Check sheet for the modelled part. Datum: model origin and axes. Units: mm. Face numbers are marked on the shaded views. A direction names the side the tool comes from. Round coordinates to 2 decimals unless told otherwise and drop trailing zeros. Order: outer loops, then holes, each group sorted by start corner. A loop starts at its lowest first (then second) coordinate and runs counter-clockwise, first axis right, second up.
Q1. Set-up check for the marked faces 1 and 2: record each of +Z, -Z, +X, -X, +Y, -Y from which the full face is reachable in a straight line by a thin tool's end or side.
Q2. Cross-section at B-B on x = 45. Record the cut outline in (y, z).
Q3. Depth check by flat-ended pin: P1, Ø3, axis at x = 15, z = -38, coming from the +Y side; P2, Ø14, axis at x = -1, z = -12.5, coming from the -Y side; P3, Ø5.5, axis at x = -18, y = -35.18, coming from the -Z side. Enter the tip coordinate at first touch or a pass-through.
Q4. Scan lines: probe 1 along X at (y, z) = (43.4, -38); probe 2 along X at (y, z) = (-35, 1); probe 3 along X at (y, z) = (32, 1.65). Record each from-to range of solid material in increasing order.
Q5. Cross-section at D-D on z = -3. Record the cut outline in (x, y), then the cut area to 3 significant figures.
Q6. Cross-section at C-C on y = 32. Record the cut outline in (x, z), then the cut area to 3 significant figures.
Q7. Cross-section at A-A on z = -31. Record the cut outline in (x, y), then the cut area to 3 significant figures.
Autodesk Inventor part; units mm, degrees
ref_plane "YZ Plane" through (0, 0, 0) normal (1, 0, 0) x (0, 1, 0)
ref_plane "XZ Plane" through (0, 0, 0) normal (0, 1, 0) x (-1, 0, 0)
ref_plane "XY Plane" through (0, 0, 0) normal (0, 0, 1) x (1, 0, 0)
sketch "Sketch3" plane through (0, 0, 0) normal (0, 0, 1) x (1, 0, 0)
  line L0 (-50, 45) -> (50, 45)
  line L1 (50, 45) -> (50, -45)
  line L2 (50, -45) -> (-50, -45)
  line L3 (-50, -45) -> (-50, 45)
  line L4 (-50, 45) -> (50, -45) construction
  line L5 (50, 45) -> (-50, -45) construction
  point P0 (0, 0)
  dimension "d4" = 100
  dimension "d5" = 90
extrude "Extrusion2" add sketch "Sketch3" along normal blind 4
sketch "Sketch4" plane through (0, 0, 4) normal (0, 0, 1) x (1, 0, 0)
  point P0 (0, 0)
sketch "Sketch5" plane through (0, 0, 4) normal (0, 0, 1) x (1, 0, 0)
  line L0 (50, 45) -> (-50, 45)
  line L1 (50, 45) -> (-50, 45)
  line L2 (-50, 45) -> (-50, 41)
  line L3 (-50, 41) -> (50, 41)
  line L4 (50, 41) -> (50, 45)
  point P0 (0, 0)
  dimension "d8" = 4
  dimension "d9" = 100
extrude "Extrusion3" add sketch "Sketch5" against normal blind 50
sketch "Sketch6" plane through (0, 0, 4) normal (0, 0, 1) x (1, 0, 0)
  line L0 (18, -31.18) -> (-18, -31.18)
  line L1 (-18, -31.18) -> (-18, 31.18)
  line L2 (-18, 31.18) -> (18, 31.18)
  line L3 (18, 31.18) -> (18, -31.18)
  line L4 (18, -31.18) -> (-18, 31.18) construction
  line L5 (-18, -31.18) -> (18, 31.18) construction
  circle A0 centre (-18, 31.18) radius 1.75
  circle A1 centre (18, 31.18) radius 1.75
  circle A2 centre (-18, -31.18) radius 1.75
  circle A3 centre (18, -31.18) radius 1.75
  line L6 (50, 45) -> (-50, 45)
  line L7 (0, 45) -> (0, -4)
  line L8 (-18, -35.18) -> (18, -35.18)
  line L9 (18, -35.18) -> (18, 27.18)
  line L10 (18, 27.18) -> (-18, 27.18)
  line L11 (-18, 27.18) -> (-18, -35.18)
  line L12 (-18, -35.18) -> (18, 27.18) construction
  line L13 (18, -35.18) -> (-18, 27.18) construction
  circle A4 centre (18, 27.18) radius 1.75
  circle A5 centre (-18, 27.18) radius 1.75
  circle A6 centre (18, -35.18) radius 1.75
  circle A7 centre (-18, -35.18) radius 1.75
  point P0 (0, 0)
  dimension "d14" = 3.5
  dimension "d15" = 3.5
  dimension "d16" = 3.5
  dimension "d17" = 3.5
  dimension "d89" = 49
  dimension "d90" = 62.36
  dimension "d91" = 3.5
  dimension "d92" = 3.5
  dimension "d93" = 3.5
  dimension "d94" = 3.5
extrude "Extrusion4" cut sketch "Sketch6" against normal blind 50 contours A5 L1 | L1 L10 A5 | A7 L8 L11 | L11 L8 A7 | A4 L10 L3 | L3 A4 | A6 L8 L9 | L9 L8 A6 | L1 A5 L10 | L10 A4 L3
sketch "Sketch7" plane through (0, 0, 4) normal (0, 0, 1) x (1, 0, 0)
  line L0 (31.18, -18) -> (-31.18, -18)
  line L1 (-31.18, -18) -> (-31.18, 18)
  line L2 (-31.18, 18) -> (31.18, 18)
  line L3 (31.18, 18) -> (31.18, -18)
  line L4 (31.18, -18) -> (-31.18, 18) construction
  line L5 (-31.18, -18) -> (31.18, 18) construction
  circle A0 centre (-31.18, 18) radius 1.75
  circle A1 centre (31.18, 18) radius 1.75
  circle A2 centre (-31.18, -18) radius 1.75
  circle A3 centre (31.18, -18) radius 1.75
  line L6 (50, 45) -> (-50, 45)
  line L7 (0, 45) -> (0, -4)
  line L8 (-31.18, -22) -> (31.18, -22)
  line L9 (31.18, -22) -> (31.18, 14)
  line L10 (31.18, 14) -> (-31.18, 14)
  line L11 (-31.18, 14) -> (-31.18, -22)
  line L12 (-31.18, -22) -> (31.18, 14) construction
  line L13 (31.18, -22) -> (-31.18, 14) construction
  circle A4 centre (31.18, 14) radius 1.75
  circle A5 centre (-31.18, 14) radius 1.75
  circle A6 centre (31.18, -22) radius 1.75
  circle A7 centre (-31.18, -22) radius 1.75
  point P0 (0, 0)
  dimension "d20" = 62.36
  dimension "d21" = 36
  dimension "d22" = 3.5
  dimension "d23" = 3.5
  dimension "d24" = 3.5
  dimension "d25" = 3.5
  dimension "d95" = 49
  dimension "d96" = 36
  dimension "d97" = 3.5
  dimension "d98" = 3.5
  dimension "d99" = 3.5
  dimension "d100" = 3.5
extrude "Extrusion5" cut sketch "Sketch7" against normal blind 50 contours A5 L1 | L1 L10 A5 | A7 L8 L11 | L11 L8 A7 | A4 L10 L3 | L3 A4 | A6 L8 L9 | L9 L8 A6 | L1 A5 L10 | L10 A4 L3
sketch "Sketch8" plane through (0, 0, 4) normal (0, 0, 1) x (1, 0, 0)
  line L0 (50, 45) -> (-50, 45)
  line L1 (0, 45) -> (0, -4)
  circle A0 centre (0, -4) radius 25
  point P0 (0, 0)
  dimension "d101" = 49
  dimension "d102" = 50
extrude "Extrusion6" cut sketch "Sketch8" against normal blind 43.6625
sketch "Sketch9" plane through (-50, 45, 4) normal (0, 1, 0) x (1, 0, 0)
  line L0 (0, 50) -> (0, 0)
  line L1 (100, 0) -> (0, 0)
  line L2 (0, 0) -> (35, 0)
  line L3 (35, 0) -> (35, 7)
  line L4 (35, 7) -> (0, 7)
  line L5 (0, 7) -> (0, 0)
  circle A0 centre (35, 7) radius 1.75
  line L6 (0, 0) -> (35, 0)
  line L7 (35, 0) -> (35, 25)
  line L8 (35, 25) -> (0, 25)
  line L9 (0, 25) -> (0, 0)
  circle A1 centre (35, 25) radius 1.75
  point P0 (50, 4)
  dimension "d31" = 35
  dimension "d32" = 7
  dimension "d36" = 3.5
  dimension "d39" = 25
  dimension "d40" = 3.5
sketch "Sketch10" plane through (-50, 45, 4) normal (0, 1, 0) x (1, 0, 0)
  line L0 (100, 4) -> (100, 0)
  line L1 (100, 0) -> (0, 0)
  line L2 (100, 0) -> (65, 0)
  line L3 (65, 0) -> (65, 7)
  line L4 (65, 7) -> (100, 7)
  line L5 (100, 7) -> (100, 0)
  circle A0 centre (65, 7) radius 1.75
  line L6 (100, 0) -> (65, 0)
  line L7 (65, 0) -> (65, 25)
  line L8 (65, 25) -> (100, 25)
  line L9 (100, 25) -> (100, 0)
  line L10 (75, 0) -> (25, 0)
  circle A1 centre (65, 25) radius 1.75
  point P0 (50, 4)
  dimension "d33" = 35
  dimension "d34" = 7
  dimension "d35" = 3.5
  dimension "d37" = 25
  dimension "d38" = 3.5
sketch "Sketch11" plane through (-50, 45, 4) normal (0, 1, 0) x (1, 0, 0)
  point P0 (50, 4)
extrude "Extrusion7" cut sketch "Sketch9" against normal blind 43.6625 contours A1 L7 L8 | L8 L7 A1 | A0 L7 L4 | L4 L3 A0 | L7 A0 L3
extrude "Extrusion8" cut sketch "Sketch10" against normal blind 43.6625 contours A0 L3 L4 | L4 L7 A0 | L3 A0 L7 | A1 L7 L8 | L8 L7 A1
sketch "Sketch12" plane through (-50, 45, 4) normal (0, 1, 0) x (1, 0, 0)
  line L0 (0, 0) -> (100, 0)
  line L1 (0, 0) -> (5, 0)
  line L2 (5, 0) -> (5, 7)
  line L3 (5, 7) -> (0, 7)
  line L4 (0, 7) -> (0, 0)
  line L5 (100, 0) -> (0, 0)
  line L6 (0, 0) -> (5, 0)
  line L7 (5, 0) -> (5, 25)
  line L8 (5, 25) -> (0, 25)
  line L9 (0, 25) -> (0, 0)
  circle A0 centre (5, 7) radius 1.75
  circle A1 centre (5, 25) radius 1.75
  point P0 (50, 4)
  dimension "d45" = 5
  dimension "d46" = 7
  dimension "d47" = 25
  dimension "d48" = 3.5
  dimension "d49" = 3.5
extrude "Extrusion9" cut sketch "Sketch12" against normal blind 43.6625 contours A0 L3 L2 | L2 L7 A0 | A0 L7 L3 | A1 L7 L8 | L8 L7 A1
sketch "Sketch13" plane through (-50, 45, 4) normal (0, 1, 0) x (1, 0, 0)
  line L0 (0, 0) -> (100, 0)
  line L1 (100, 0) -> (95, 0)
  line L2 (95, 0) -> (95, 7)
  line L3 (95, 7) -> (100, 7)
  line L4 (100, 7) -> (100, 0)
  line L5 (100, 0) -> (95, 0)
  line L6 (95, 0) -> (95, 25)
  line L7 (95, 25) -> (100, 25)
  line L8 (100, 25) -> (100, 0)
  circle A0 centre (95, 25) radius 1.75
  circle A1 centre (95, 7) radius 1.75
  point P0 (50, 4)
  dimension "d52" = 5
  dimension "d53" = 7
  dimension "d54" = 25
  dimension "d55" = 3.5
  dimension "d56" = 3.5
extrude "Extrusion10" cut sketch "Sketch13" against normal blind 43.6625 contours A1 L6 L2 | L2 L3 A1 | L6 A1 L3 | A0 L7 L6 | L6 L7 A0
sketch "Sketch14" plane through (-50, 45, 4) normal (0, 1, 0) x (1, 0, 0)
  point P0 (50, 4)
sketch "Sketch15" plane through (-50, 45, 4) normal (0, 1, 0) x (1, 0, 0)
  line L0 (0, 50) -> (100, 50)
  line L1 (0, 50) -> (50, 50)
  line L2 (50, 50) -> (50, 42)
  line L3 (50, 42) -> (0, 42)
  line L4 (0, 42) -> (0, 50)
  line L5 (0, 50) -> (35, 50)
  line L6 (35, 50) -> (35, 42)
  line L7 (35, 42) -> (0, 42)
  line L8 (0, 42) -> (0, 50)
  line L9 (0, 4) -> (0, 50)
  line L10 (0, 50) -> (5, 50)
  line L11 (5, 50) -> (5, 42)
  line L12 (5, 42) -> (0, 42)
  line L13 (0, 42) -> (0, 50)
  line L14 (100, 4) -> (100, 50)
  line L15 (100, 50) -> (95, 50)
  line L16 (95, 50) -> (95, 42)
  line L17 (95, 42) -> (100, 42)
  line L18 (100, 42) -> (100, 50)
  line L19 (100, 50) -> (0, 50)
  line L20 (100, 50) -> (65, 50)
  line L21 (65, 50) -> (65, 42)
  line L22 (65, 42) -> (100, 42)
  line L23 (100, 42) -> (100, 50)
  circle A0 centre (5, 42) radius 1.75
  circle A1 centre (35, 42) radius 1.75
  circle A2 centre (65, 42) radius 1.75
  circle A3 centre (95, 42) radius 1.75
  point P0 (50, 4)
  dimension "d60" = 8
  dimension "d61" = 35
  dimension "d62" = 5
  dimension "d63" = 5
  dimension "d64" = 35
  dimension "d66" = 3.5
  dimension "d67" = 3.5
  dimension "d68" = 3.5
  dimension "d69" = 3.5
extrude "Extrusion11" cut sketch "Sketch15" against normal blind 43.6625 contours A0 L3 L11 | L11 L3 A0 | L3 A0 | A1 L3 L6 | L6 L3 A1 | L3 A1 | A2 L22 L21 | L21 L22 A2 | A3 L17 L16 | L16 L22 A3 | L17 A3 L22
sketch "Sketch16" plane through (-50, 45, 4) normal (0, 1, 0) x (1, 0, 0)
  line L0 (100, 50) -> (0, 50)
  line L1 (0, 50) -> (20, 50)
  line L2 (20, 50) -> (20, 35)
  line L3 (20, 35) -> (0, 35)
  line L4 (0, 35) -> (0, 50)
  line L5 (0, 50) -> (0, 0)
  line L6 (0, 50) -> (50, 50)
  line L7 (50, 50) -> (50, 35)
  line L8 (50, 35) -> (0, 35)
  line L9 (0, 35) -> (0, 50)
  line L10 (100, 4) -> (100, 50)
  line L11 (100, 50) -> (80, 50)
  line L12 (80, 50) -> (80, 35)
  line L13 (80, 35) -> (100, 35)
  line L14 (100, 35) -> (100, 50)
  circle A0 centre (20, 35) radius 1.75
  circle A1 centre (50, 35) radius 1.75
  circle A2 centre (80, 35) radius 1.75
  point P0 (50, 4)
  dimension "d72" = 20
  dimension "d73" = 15
  dimension "d74" = 50
  dimension "d75" = 20
  dimension "d76" = 3.5
  dimension "d77" = 3.5
  dimension "d78" = 3.5
extrude "Extrusion12" cut sketch "Sketch16" against normal blind 10 contours A2 L13 L12 | L12 L13 A2 | A1 L8 L7 | L7 L8 A1 | A0 L8 L2 | L2 L3 A0 | L8 A0 L3
sketch "Sketch17" plane through (0, 0, 4) normal (0, 0, 1) x (1, 0, 0)
  line L0 (36, -36) -> (-36, -36)
  line L1 (-36, -36) -> (-36, 36)
  line L2 (-36, 36) -> (36, 36)
  line L3 (36, 36) -> (36, -36)
  line L4 (36, -36) -> (-36, 36) construction
  line L5 (-36, -36) -> (36, 36) construction
  circle A0 centre (-36, 36) radius 1.75
  circle A1 centre (36, 36) radius 1.75
  circle A2 centre (36, -36) radius 1.75
  circle A3 centre (-36, -36) radius 1.75
  line L6 (50, 45) -> (-50, 45)
  line L7 (0, 45) -> (0, -4)
  line L8 (-36, -40) -> (36, -40)
  line L9 (36, -40) -> (36, 32)
  line L10 (36, 32) -> (-36, 32)
  line L11 (-36, 32) -> (-36, -40)
  line L12 (-36, -40) -> (36, 32) construction
  line L13 (36, -40) -> (-36, 32) construction
  circle A4 centre (36, 32) radius 1.75
  circle A5 centre (36, -40) radius 1.75
  circle A6 centre (-36, -40) radius 1.75
  circle A7 centre (-36, 32) radius 1.75
  point P0 (0, 0)
  dimension "d81" = 72
  dimension "d82" = 72
  dimension "d83" = 3.5
  dimension "d84" = 3.5
  dimension "d85" = 3.5
  dimension "d86" = 3.5
  dimension "d103" = 49
  dimension "d104" = 72
  dimension "d105" = 3.5
  dimension "d106" = 3.5
  dimension "d107" = 3.5
  dimension "d108" = 3.5
extrude "Extrusion13" cut sketch "Sketch17" against normal blind 10 contours A7 L1 | L1 L10 A7 | A6 L8 L11 | L11 L8 A6 | A4 L10 L3 | L3 A4 | A5 L8 L9 | L9 L8 A5 | L1 A7 L10 | L10 A4 L3
properties part number "ousterholderm600V2"
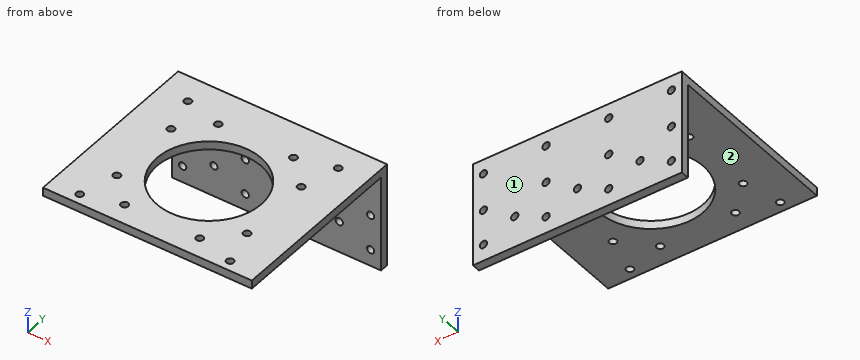
Results found:
1. face 1: +Z, -Z, +X, -X, +Y
1. face 2: -Z, +X, -X, -Y
2. outline: (-45, 0) - (41, 0) - (41, -1.25) - (45, -1.25) - (45, 4) - (-45, 4) - close; (41, -46) - (45, -46) - (45, -39.75) - (41, -39.75) - close; (41, -36.25) - (45, -36.25) - (45, -22.75) - (41, -22.75) - close; (41, -19.25) - (45, -19.25) - (45, -4.75) - (41, -4.75) - close
3. P1: passes through
3. P2: stops at y = 41
3. P3: stops at z = 0
4. probe 1: x = -50 to -46.75, -43.25 to -16.75, -13.25 to 13.25, 16.75 to 43.25, 46.75 to 50
4. probe 2: x = -50 to -19.74, -16.26 to 16.26, 19.74 to 50
4. probe 3: x = -50 to -37.75, -34.25 to 34.25, 37.75 to 50
5. outline: (-50, 41) - (-46.75, 41) - (-46.75, 45) - (-50, 45) - close; (-43.25, 41) - (-16.75, 41) - (-16.75, 45) - (-43.25, 45) - close; (-13.25, 41) - (13.25, 41) - (13.25, 45) - (-13.25, 45) - close; (16.75, 41) - (43.25, 41) - (43.25, 45) - (16.75, 45) - close; (46.75, 41) - (50, 41) - (50, 45) - (46.75, 45) - close
5. area: 344 mm2
6. outline: (-50, 0) - (-37.75, 0) - (-37.75, 4) - (-50, 4) - close; (-34.25, 0) - (34.25, 0) - (34.25, 4) - (-34.25, 4) - close; (37.75, 0) - (50, 0) - (50, 4) - (37.75, 4) - close
6. area: 372 mm2
7. outline: (-50, 41) - (-31.75, 41) - (-31.75, 45) - (-50, 45) - close; (-28.25, 41) - (-1.75, 41) - (-1.75, 45) - (-28.25, 45) - close; (1.75, 41) - (28.25, 41) - (28.25, 45) - (1.75, 45) - close; (31.75, 41) - (50, 41) - (50, 45) - (31.75, 45) - close
7. area: 358 mm2
